Autodesk Inventor part; units mm, degrees
ref_plane "YZ Plane" through (0, 0, 0) normal (1, 0, 0) x (0, 1, 0)
ref_plane "XZ Plane" through (0, 0, 0) normal (0, 1, 0) x (-1, 0, 0)
ref_plane "XY Plane" through (0, 0, 0) normal (0, 0, 1) x (1, 0, 0)
sketch "Sketch1" plane through (0, 0, 0) normal (0, 1, 0) x (-1, 0, 0)
  arc A0 (11.5434, 7) -> (11.5434, -7) centre (0, 0) ccw
  line L0 (13.5, 0) -> (20.5, 0) construction
  line L1 (13.5, -7) -> (13.5, 7)
  line L2 (13.5, 7) -> (11.5434, 7)
  line L3 (13.5, -7) -> (11.5434, -7)
  dimension "d0" = 27
  dimension "d1" = 7
  dimension "d3" = 14
extrude "Extrusion1" add sketch "Sketch1" along normal blind 15
sketch "Sketch2" plane through (0, 15, 0) normal (0, 1, 0) x (1, 0, 0)
  circle A0 centre (0, 0) radius 11
  dimension "d6" = 22
extrude "Extrusion2" add sketch "Sketch2" along normal blind 2
sketch "Sketch3" plane through (0, 17, 0) normal (0, 1, 0) x (1, 0, 0)
  circle A0 centre (0, 0) radius 10
  dimension "d9" = 20
extrude "Extrusion3" add sketch "Sketch3" along normal blind 2
sketch "Sketch4" plane through (0, 19, 0) normal (0, 1, 0) x (1, 0, 0)
  circle A0 centre (0, 0) radius 10.5
  dimension "d12" = 21
extrude "Extrusion4" add sketch "Sketch4" along normal blind 16
fillet "Fillet1" radius 1 1 edges at (-10, 17, 0)
chamfer "Chamfer1" distance 0.5 angle 45 2 edges at (-10, 19, 0) (-10.5, 19, 0)
fillet "Fillet2" radius 0.5 1 edges at (-10.5, 35, 0)
thread "Thread1"
sketch "Sketch5" plane through (-13.5, 0, -7) normal (-1, 0, 0) x (0, 0, 1)
  point P0 (7, 0)
sketch "Sketch6" plane through (0, 0, 0) normal (0, -1, 0) x (1, 0, 0)
  circle A0 centre (0, 0) radius 7.5
  dimension "d22" = 15
extrude "Extrusion5" cut sketch "Sketch6" against normal blind 25
sketch "Sketch7" plane through (-13.5, 0, -7) normal (-1, 0, 0) x (0, 0, 1)
  circle A0 centre (7, 7.5) radius 4.5
  point P0 (7, 0)
  dimension "d25" = 9
extrude "Extrusion6" cut sketch "Sketch7" against normal blind 18
thread "Thread2"
sketch "Sketch8" plane through (0, 35, 0) normal (0, 1, 0) x (1, 0, 0)
  circle A0 centre (0, 0) radius 6.5
  dimension "d30" = 13
extrude "Extrusion7" cut sketch "Sketch8" against normal blind 18
sketch "Sketch9" plane through (0, 35, 0) normal (0, 1, 0) x (1, 0, 0)
  point P0 (0, 0)
properties part number "prednji deo" material "ABS Plastic"
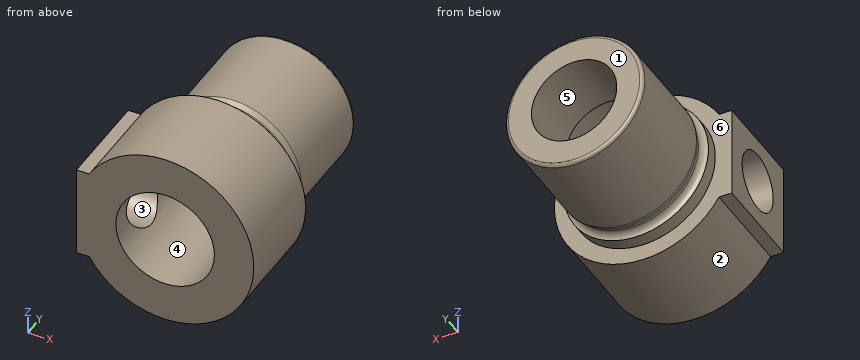
Design review of the part built by this model. Coordinates are the model's own, in mm. Face numbers are marked on the shaded views. A direction names the side the tool comes from. Coordinates: 2 decimals unless noted, no trailing zeros. Order: outer loops, then holes, each group sorted by start corner. A loop starts at its lowest first (then second) coordinate and runs counter-clockwise, first axis right, second up.
1) Clearance check with flat-ended pins moving along their axes: pin 1 (1 mm diameter, centred on y = 4.5, z = -2, fed in from -X); pin 2 (1 mm diameter, centred on x = 9, y = 20.5, fed in from -Z); pin 3 (0.6 mm diameter, centred on x = -13, y = 8, fed in from +Z). State where each tip first meets the part, or that it passes through.
2) Take a section at C-C, the plane y = 7.5. Give the boundary of the cut face in (x, z).
3) Wall thickness on line 1 along Y through (x, z) = (-12, 0); line 2 along Z through (x, y) = (0, 11); line 3 along Z through (x, y) = (0, 18.5): over which ranges is each line inside the solid? List them lowest first.
4) Take a section at A-A, the plane z = 0. State how many separate pieces and enclosed holes the cut face has, and give its area (3 significant figures).
5) Mouldability with a two-part tool opening along Y and no side actions: class the marked faces 1, 2 and 3 as +Y half, -Y half, draft (parallel to the pull), parting line (faces both ways), or undercut.
6) For the marked faces 4, 5 and 6, list the 3-axis set-ups (+Z, -Z, +X, -X, +Y, -Y) from which the entire face can be reached by the end or side of a thin tool; tool diameter is ignored.
7) Take a section at D-D, the plane y = 28.5. Give the boundary of the cut face in (x, z), and give its area (3 significant figures).
Returned:
1. pin 1: stops at x = 7.07
1. pin 2: stops at z = -6.16
1. pin 3: stops at z = 7
2. outline: (-13.5, -7) - (-11.54, -7) arc R13.5 ccw (long way) to (-11.54, 7) - (-13.5, 7) - (-13.5, 4.5) - (-6, 4.5) arc R7.5 cw (long way) to (-6, -4.5) - (-13.5, -4.5) - close
3. line 1: y = 0 to 3, 12 to 15
3. line 2: z = -13.5 to -7.5, 7.5 to 13.5
3. line 3: z = -10 to -7.5, 7.5 to 10
4. separate pieces: 3
4. enclosed holes: 0
4. area: 266 mm2
5. face 1: +Y half
5. face 2: draft
5. face 3: undercut
6. face 4: -Y
6. face 5: +Y, -Y
6. face 6: +Y
7. outline: circle Ø21 at (0, 0); hole circle Ø13 at (0, 0)
7. area: 214 mm2
